For this review, take the finished solid that the model builds, in its own axes (mm). Face numbers are marked on the shaded views. A direction names the side the tool comes from. Give positions to 0.01 mm unless a question says otherwise; leave off trailing zeros. Order: outer loops, then holes, each group sorted by start corner. A loop starts at its lowest first (then second) coordinate and runs counter-clockwise, first axis right, second up. Notation, with made-up numbers: M 72,17.5 L 123,17.5 A9 ccw 123,27.5 Z; hole C 47,1 d5. An arc over 180 degrees is marked long. Answer as CSV lines item,"result". Start each with the question number.
1. Mouldability with a two-part tool opening along Y and no side actions: class the marked faces 1 and 2 as pulls with the +Y half, pulls with the -Y half, needs draft (parallel to the pull), parting line crosses it, or undercut.
2. We need section D-D, the plane y = 8.25. Give the boundary of the cut face in (x, z), and give its area (3 significant figures).
3. Clearance check with flat-ended pins moving along their axes: P1, Ø5, axis at x = 6, y = -8.5, coming from the +Z side; P2, Ø1, axis at x = -4.5, z = 4, coming from the +Y side; P3, Ø3, axis at y = 7, z = 2, coming from the +X side; P4, Ø3, axis at x = 9, z = 0, coming from the +Y side. State where each tip first meets the part, or that it passes through.
4. For line 1 along X through (y, z) = (4.5, 6.75); line 2 along Y through (x, z) = (0.75, 2); line 3 along Z through (x, y) = (6.25, -10), list the stretches that pass through material, from the lowest coordinate up.
5. We need section A-A, the plane x = 0. Give the boundary of the cut face in (y, z) (1 decimal), and give its area (3 significant figures).
6. We need section C-C, the plane z = 2. Give the boundary of the cut face in (x, y), and give its area (3 significant figures).
7. Machinability: for the marked faces 3 and 4, which of the approach directions +Z, -Z, +X, -X, +Y, -Y give a long, thin tool a straight path to every point of the face, cutting with its end or side? Answer none if there is none.
from build123d import *

# Parameters (mm, degrees)
F0_R     = 12.7
F0_R_2   = 8.636
F1_DEPTH = 2.54
F2_DEPTH = 7.62


with BuildPart() as f1:
    # F0 (on Top) → F1 (new body)
    with BuildSketch(Plane.XY):
        Circle(F0_R)
        Circle(F0_R_2, mode=Mode.SUBTRACT)
        Circle(F0_R_2)
    extrude(amount=-F1_DEPTH)

    # F0 (on Top) → F2 (join)
    with BuildSketch(Plane.XY):
        Circle(F0_R_2)
    extrude(amount=F2_DEPTH)

    # F3 (on Front) → F4 (revolve, cut)
    with BuildSketch(Plane.XZ):
        with BuildLine():
            Line((0, 14.949476), (0, 0.979476))
            ThreePointArc((0, 0.979476), (6.985, 7.964476), (0, 14.949476))
        make_face()
    revolve(axis=Axis((0, 0, 5.221219), (0, 0, -1)), mode=Mode.SUBTRACT)


solid = f1.part
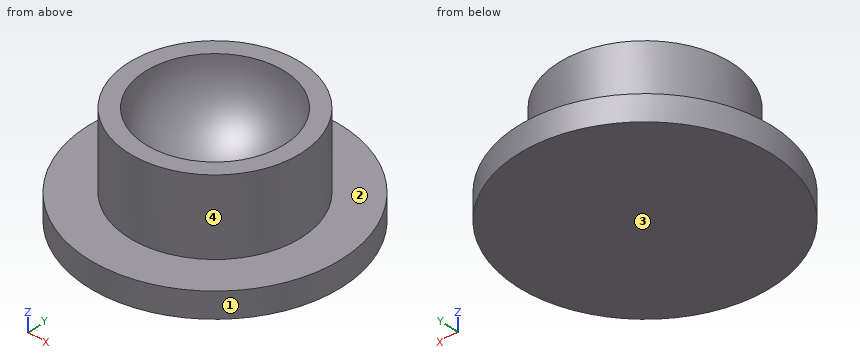
Result set:
1,face 1,"parting line crosses it"
1,face 2,"needs draft"
2,outline,"M -9.66,-2.54 L 9.66,-2.54 L 9.66,0 L 2.55,0 L 2.55,7.62 L -2.55,7.62 L -2.55,0 L -9.66,0 Z"
2,area,"88.0 mm2"
3,P1,"z = 7.62"
3,P2,"y = 7.65"
3,P3,"x = 6.66"
3,P4,"y = 10.25"
4,line 1,"-7.37 to -5.2, 5.2 to 7.37"
4,line 2,"-8.6 to -3.56, 3.56 to 8.6"
4,line 3,"-2.54 to 0"
5,outline,"M -12.7,-2.5 L 12.7,-2.5 L 12.7,0 L 8.6,0 L 8.6,7.6 L 7,7.6 A7 cw -7,7.6 L -8.6,7.6 L -8.6,0 L -12.7,0 Z"
5,area,"124 mm2"
6,outline,"C 0,0 d17.27; hole C 0,0 d7.27"
6,area,"193 mm2"
7,face 3,"-Z, +X, -X, +Y, -Y"
7,face 4,"+Z"
